```python
from build123d import *

# Parameters (mm, degrees)
BOSS_EXTRUDE1_DEPTH = 20
SKETCH2_R           = 1.65
CUT_EXTRUDE1_DEPTH  = 7
SKETCH3_R           = 1.4
CUT_EXTRUDE2_DEPTH  = 27


with BuildPart() as part:
    # Sketch1 → Boss-Extrude1 (new body)
    with BuildSketch(Plane.XY):
        with BuildLine():
            Line((0, 123.395512055), (0, 108.395512055))
            Line((0, 108.395512055), (-7.2, 108.395512055))
            Line((-7.2, 108.395512055), (-7.2, 123.395512055))
            Line((-7.2, 123.395512055), (-14.2, 123.395512055))
            add(Edge.make_bspline(
                [(-14.2, 123.395512055), (-23.530576474, 117.205565192), (-38.446210931, 109.915945525), (-66.691471381, 105.395512055), (-83, 105.395512055)],
                knots=[0, 0, 0, 0, 0.267223526, 1, 1, 1, 1], degree=3))
            Line((-83, 105.395512055), (-83, 98.395512055))
            Line((-83, 98.395512055), (7, 98.395512055))
            Line((7, 98.395512055), (7, 123.395512055))
            Line((7, 123.395512055), (0, 123.395512055))
        make_face()
    extrude(amount=BOSS_EXTRUDE1_DEPTH)

    # Sketch2 → Cut-Extrude1 (cut)
    with BuildSketch(Plane(origin=(7, 0, 0), x_dir=(0, 0, -1), z_dir=(1, 0, 0))):
        with Locations((-15, 117.395512055)):
            Circle(SKETCH2_R)
        with Locations((-5, 117.395512055)):
            Circle(SKETCH2_R)
    extrude(amount=-CUT_EXTRUDE1_DEPTH, mode=Mode.SUBTRACT)

    # Sketch3 → Cut-Extrude2 (cut)
    with BuildSketch(Plane(origin=(-7.2, 0, 0), x_dir=(0, 0, -1), z_dir=(1, 0, 0))):
        with Locations((-15, 117.395512055)):
            Circle(SKETCH3_R)
        with Locations((-5, 117.395512055)):
            Circle(SKETCH3_R)
    extrude(amount=-CUT_EXTRUDE2_DEPTH, mode=Mode.SUBTRACT)


solid = part.part
```
The model under review builds one solid part; all positions refer to its coordinate system, in mm. A direction names the side the tool comes from. Round coordinates to 2 decimals unless told otherwise and drop trailing zeros. Loops run counter-clockwise (first coordinate to the right, second up) from the corner with the lowest first, then second, coordinate; pieces in that order, holes last. Notation, with made-up numbers: (81.5, 18.25) - (114.5, 18.25) arc R19 ccw to (114.5, 23.25) - close; hole circle Ø7 at (79.5, 6). An arc over 180 degrees is marked (long way). Write each question's results on one line, items separated by ' | '. Start each with the question number.
Q1. Take a section at B-B on z = 5. Give the number of separate pieces and of enclosed holes in the cut face, plus the area to 3 significant figures.
Q2. Insertion check: P1, Ø10, axis at x = -13.5, y = 101.5, coming from the -Z side; P2, Ø5, axis at y = 120.5, z = 3.5, coming from the -X side; P3, Ø2, axis at y = 117.4, z = 15, coming from the +X side; P4, Ø5.5, axis at y = 117.4, z = 5, coming from the -X side. Each pin has a flat end and moves straight along its axis. Give the tip position at first contact, or say it passes through.
Q3. Draft analysis for pull direction Y (two halves, no side actions). For faces 4 (the flat face through (0, 116, 10)), 5 (the flat face through (-11, 123.396, 10)), 6 (the cylindrical face through (3.549, 115.785, 15.358)), state which applies: pulls with the +Y half, pulls with the -Y half, needs draft (parallel to the pull), parting line crosses it, or undercut.
Q4. Tool access review of faces 1 (the flat face through (-39, 98.396, 10)), 2 (the cylindrical face through (3.549, 115.785, 5.358)), 3 (the flat face through (-4, 108.396, 10)): name each direction out of +Z, -Z, +X, -X, +Y, -Y from which nothing blocks a thin tool from reaching the whole face with its end or side.
Q5. Wall thickness on line 1 along Y through (x, z) = (1.5, 15); line 2 along Z through (x, y) = (-8, 117); line 3 along Y through (x, z) = (-7, 18.25): over which ranges is each line inside the solid? List them lowest first. Write a range as [from, to].
Q6. Take a section at A-A on x = -3.5. Give the boundary of the cut face in (y, z).
Data:
1) separate pieces: 3 | enclosed holes: 0 | area: 1,200 mm²
2) P1: stops at z = 0 | P2: stops at x = -22.79 | P3: passes through | P4: stops at x = -29.47
3) face 4: needs draft | face 5: pulls with the +Y half | face 6: undercut
4) face 1: +Z, -Z, +X, -X, -Y | face 2: +X | face 3: +Z, -Z, +Y
5) line 1: y = [98.4, 115.75], [119.05, 123.4] | line 2: z = [0, 3.66], [6.34, 13.66], [16.34, 20] | line 3: y = [98.4, 108.4]
6) outline: (98.4, 0) - (108.4, 0) - (108.4, 20) - (98.4, 20) - close
